Read the model definition and answer for the solid it produces. Units are mm, in the model's axes. Coordinates: 2 decimals unless noted, no trailing zeros. Write each loop counter-clockwise with the first axis right and the second up, starting at its lowest first coordinate (ties: lowest second). Pieces come first, ordered by that corner, then holes. Notation, with made-up numbers: (76, -27.75) -> (118, -27.75) arc R22 ccw to (118, -18.75) -> close; hole circle Ø7 at (75, 8). An arc over 180 degrees is marked (long way). One line per item, written item: value. Start each with the question number.
1. Find section A-A, the plane y = 0. Write down the section's boundary in (x, z).
2. Find section C-C, the plane z = 1.7. Write down the section's boundary in (x, y), and give its area (3 significant figures).
3. Given P1, Ø2, axis at x = 32.5, z = 3, coming from the -Y side; P2, Ø1.5, axis at x = 41.5, z = 3, coming from the -Y side, each flat-ended and moving along its own axis, determine where each tip first touches the part or whether it passes through.
4. Find section D-D, the plane x = 23.5. Write down the section's boundary in (y, z), and give its area (3 significant figures).
5. Consider line 1 along X through (y, z) = (31, 0.25); line 2 along X through (y, z) = (-39, 2.9); line 3 along Y through (x, z) = (-2.5, 0.55). Determine where each line is inside the solid, lowest interval first.
```python
from build123d import *

# Parameters (mm, degrees)
SKICA1_R                = 5
P_IDAT_VYSUNUT_M1_DEPTH = 5


with BuildPart() as part:
    # Skica1 → Přidat vysunutím1 (new body)
    with BuildSketch(Plane.XY):
        with BuildLine():
            Line((11.954171039, 19.378792599), (43.773975828, 51.198598116))
            ThreePointArc((43.773975828, 51.198598116), (45.525986921, 55.694516194), (43.400986545, 60.026628339))
            ThreePointArc((43.400986545, 60.026628339), (5.05e-07, 42.500001775), (-43.400985944, 60.026627326))
            ThreePointArc((-43.400985944, 60.026627326), (-45.525987252, 55.694514886), (-43.77397602, 51.198596137))
            Line((-43.77397602, 51.198596137), (-11.954170503, 19.378791347))
            ThreePointArc((-11.954170503, 19.378791347), (-11.954171755, 11.954171481), (-19.378791621, 11.95417006))
            Line((-19.378791621, 11.95417006), (-51.198597038, 43.77397475))
            ThreePointArc((-51.198597038, 43.77397475), (-55.694514292, 45.525985877), (-60.026626197, 43.400986726))
            ThreePointArc((-60.026626197, 43.400986726), (-42.5, -1.49e-07), (-60.026626405, -43.400986941))
            ThreePointArc((-60.026626405, -43.400986941), (-55.694514208, -45.525987235), (-51.198596158, -43.773976041))
            Line((-51.198596158, -43.773976041), (-19.378791368, -11.954170524))
            ThreePointArc((-19.378791368, -11.954170524), (-11.954170343, -11.954171064), (-11.954170848, -19.378792089))
            Line((-11.954170848, -19.378792089), (-43.773975638, -51.198597606))
            ThreePointArc((-43.773975638, -51.198597606), (-45.52598669, -55.694515634), (-43.400986372, -60.026627739))
            ThreePointArc((-43.400986372, -60.026627739), (-7.5e-08, -42.500001775), (43.400986138, -60.026627946))
            ThreePointArc((43.400986138, -60.026627946), (45.525987031, -55.694515759), (43.773976041, -51.198597357))
            Line((43.773976041, -51.198597357), (11.954170524, -19.378792567))
            ThreePointArc((11.954170524, -19.378792567), (11.954170439, -11.954170166), (19.378792841, -11.954170081))
            Line((19.378792841, -11.954170081), (51.198597688, -43.773974201))
            ThreePointArc((51.198597688, -43.773974201), (55.694514488, -45.525985242), (60.026626197, -43.400986726))
            ThreePointArc((60.026626197, -43.400986726), (42.5, 8.27e-07), (60.026627347, 43.400987917))
            ThreePointArc((60.026627347, 43.400987917), (55.694515153, 45.525988194), (51.198597116, 43.773976998))
            Line((51.198597116, 43.773976998), (19.378792326, 11.954171481))
            ThreePointArc((19.378792326, 11.954171481), (11.954171123, 11.954171397), (11.954171039, 19.378792599))
        make_face()
        Circle(SKICA1_R, mode=Mode.SUBTRACT)
    extrude(amount=P_IDAT_VYSUNUT_M1_DEPTH)


solid = part.part
```
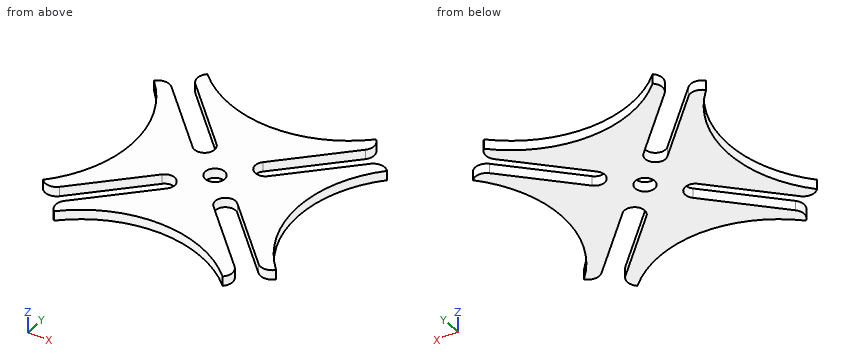
Answer block:
1. outline: (-42.5, 0) -> (-5, 0) -> (-5, 5) -> (-42.5, 5) -> close; (5, 0) -> (42.5, 0) -> (42.5, 5) -> (5, 5) -> close
2. outline: (-60.03, -43.4) arc R6 ccw to (-51.2, -43.77) -> (-19.38, -11.95) arc R5.25 cw to (-11.95, -19.38) -> (-43.77, -51.2) arc R6 ccw to (-43.4, -60.03) arc R62.5 cw to (43.4, -60.03) arc R6 ccw to (43.77, -51.2) -> (11.95, -19.38) arc R5.25 cw to (19.38, -11.95) -> (51.2, -43.77) arc R6 ccw to (60.03, -43.4) arc R62.5 cw to (60.03, 43.4) arc R6 ccw to (51.2, 43.77) -> (19.38, 11.95) arc R5.25 cw to (11.95, 19.38) -> (43.77, 51.2) arc R6 ccw to (43.4, 60.03) arc R62.5 cw to (-43.4, 60.03) arc R6 ccw to (-43.77, 51.2) -> (-11.95, 19.38) arc R5.25 cw to (-19.38, 11.95) -> (-51.2, 43.77) arc R6 ccw to (-60.03, 43.4) arc R62.5 cw to start; hole circle Ø10 at (0, 0)
2. area: 7,220 mm2
3. P1: stops at y = -52.24
3. P2: stops at y = -58.94
4. outline: (-47.09, 0) -> (-30.92, 0) -> (-30.92, 5) -> (-47.09, 5) -> close; (-16.08, 0) -> (16.08, 0) -> (16.08, 5) -> (-16.08, 5) -> close; (30.92, 0) -> (47.09, 0) -> (47.09, 5) -> (30.92, 5) -> close
4. area: 322 mm2
5. line 1: x = -50.73 to -38.42, -23.58 to 23.58, 38.42 to 50.73
5. line 2: x = -56.16 to -46.42, -31.58 to 31.58, 46.42 to 56.16
5. line 3: y = -42.55 to -4.33, 4.33 to 42.55
